Check sheet for the modelled part. Datum: model origin and axes. Units: mm. A direction names the side the tool comes from. Round coordinates to 2 decimals unless told otherwise and drop trailing zeros. Loops run counter-clockwise (first coordinate to the right, second up) from the corner with the lowest first, then second, coordinate; pieces in that order, holes last. Notation, with made-up numbers: (27, 15.5) -> (52, 15.5) arc R14 cw to (52, 34.5) -> close; hole circle Ø4 at (2, 63). An arc over 180 degrees is marked (long way). One line per question, with ' | ' between items.
```python
from build123d import *

# Parameters (mm, degrees)
SKETCH1_W      = 140
SKETCH1_H      = 150
EXTRUDE1_DEPTH = 15
EXTRUDE2_DEPTH = 150
EXTRUDE3_REACH = 92


with BuildPart() as part:
    # Sketch1 → Extrude1 (new body)
    with BuildSketch(Plane(origin=(0, 0, 0), x_dir=(1, 0, 0), z_dir=(0, 1, 0))):
        with Locations((-70, 75)):
            Rectangle(SKETCH1_W, SKETCH1_H)
    extrude(amount=EXTRUDE1_DEPTH)

    # Sketch2 → Extrude2 (add)
    with BuildSketch(Plane.XY):
        Polygon((-25, 15), (-25, 30), (-50, 30), (-50, 45), (-115, 45), (-115, 96.25), (0, 125), (0, 135), (-140, 100), (-140, 15), align=None)
    extrude(amount=-EXTRUDE2_DEPTH)

    # Extrude3: up to this plane
    extrude3_end = Plane(origin=(-115, 96.25, -150), z_dir=(0.242535625, -0.9701425, 0))
    # Sketch3 → Extrude3 (add, up to the surface)
    with BuildSketch(Plane(origin=(0, 45, 0), x_dir=(1, 0, 0), z_dir=(0, 1, 0)), mode=Mode.PRIVATE) as extrude3_sk1:
        Polygon((-115, 150), (-75, 125), (-75, 25), (-115, 0), align=None)
    extrude3_tool1 = split(extrude(extrude3_sk1.sketch, amount=EXTRUDE3_REACH, mode=Mode.PRIVATE), bisect_by=extrude3_end, keep=Keep.BOTH, mode=Mode.PRIVATE)
    add(extrude3_tool1.solids().sort_by_distance((-96.333333, 45, -75))[0])


solid = part.part
```
(1) Sectioned sample at C-C, the plane y = 81. Record the cut outline in (x, z), and give its area (3 significant figures).
Answer:
outline: (-140, -150) -> (-115, -150) -> (-75, -125) -> (-75, -25) -> (-115, 0) -> (-140, 0) -> close | area: 8,750 mm2
(2) Go/stop test with flat-tipped pins: pin 1 (8 mm diameter, centred on x = -53, z = -123, fed in from +Y); pin 2 (16.5 mm diameter, centred on y = 39.5, z = -107.5, fed in from +X); pin 3 (7.5 mm diameter, centred on x = -35, z = -57.5, fed in from +Y). Record where each tip stops, or that it passes through.
Answer:
pin 1: stops at y = 122.75 | pin 2: stops at x = -50 | pin 3: stops at y = 127.19
(3) Set-up check for faces 4 (the face through (-37, 30, -74)), 5 (the face through (-95.28, 75.196, -137.675)), 6 (the face through (0, 7, -74)), 7 (the face through (-94.72, 75.196, -12.675)), 8 (the face through (-87, 38, 0)): record each of +Z, -Z, +X, -X, +Y, -Y from which the full face is reachable in a straight line by a thin tool's end or side.
Answer:
face 4: +Z, -Z, +X | face 5: -Z, +X | face 6: +Z, -Z, +X, +Y, -Y | face 7: +Z, +X | face 8: +Z, +X, -X, +Y, -Y
(4) Sectioned sample at B-B, the plane z = -65.5. Record the cut outline in (x, y).
Answer:
outline: (-140, 0) -> (0, 0) -> (0, 15) -> (-25, 15) -> (-25, 30) -> (-50, 30) -> (-50, 45) -> (-75, 45) -> (-75, 106.25) -> (0, 125) -> (0, 135) -> (-140, 100) -> close
(5) Sectioned sample at A-A, the plane x = -19. Record the cut outline in (y, z), and give its area (3 significant figures).
Answer:
outline: (0, -150) -> (15, -150) -> (15, 0) -> (0, 0) -> close; (120.25, -150) -> (130.25, -150) -> (130.25, 0) -> (120.25, 0) -> close | area: 3,750 mm2
(6) Scan lines: probe 1 along Y at (x, z) = (-78.5, -142) (3 decimals); probe 2 along X at (y, z) = (21, -45); probe 3 along X at (y, z) = (91.5, -106.5). Record each from-to range of solid material in increasing order.
Answer:
probe 1: y = 0 to 45, 105.375 to 115.375 | probe 2: x = -140 to -25 | probe 3: x = -140 to -75
(7) Mould release check, pull along Y, two halves, no side actions. Record for faces 1 (the face through (-13, 15, -76)), 2 (the face through (-69.02, 117.745, -73.95)), 3 (the face through (-71, 0, -76)): +Y half, -Y half, draft (parallel to the pull), parting line (faces both ways), or undercut.
Answer:
face 1: undercut | face 2: +Y half | face 3: -Y half
(8) Sectioned sample at D-D, the plane x = -90. Record the cut outline in (y, z) (3 decimals).
Answer:
outline: (0, -150) -> (45, -150) -> (45, -134.375) -> (102.5, -134.375) -> (102.5, -150) -> (112.5, -150) -> (112.5, 0) -> (102.5, 0) -> (102.5, -15.625) -> (45, -15.625) -> (45, 0) -> (0, 0) -> close
